Source: CAD feature listing. Evaluate the final solid. Frame: model axes, mm. A direction names the side the tool comes from. Give positions to 0.01 mm unless a question says otherwise; leave off trailing zeros. Write each loop counter-clockwise with the first axis right and the second up, starting at its lowest first coordinate (ties: lowest second). Pieces come first, ordered by that corner, then holes. Notation, with made-up numbers: (86.5, -35.75) -> (122.5, -35.75) arc R11 ccw to (122.5, -25.75) -> close; hole circle Ø3 at (35.5, -16). An arc over 180 degrees is marked (long way). Use a Markdown table: item, result. Add a question column.
```python
from build123d import *

# Parameters (mm, degrees)
EXTRUDE_1_DEPTH           = 25
SKETCH_4_R                = 2.5
EXTRUDE_2_DEPTH           = 7
M5X0_8_TAPPED_HOLE1_D     = 4.2
M5X0_8_TAPPED_HOLE1_DEPTH = 14
M5X0_8_TAPPED_HOLE1_TIP   = 1.2618073


with BuildPart() as part:
    # 草圖1 → 填料-伸長1 (new body)
    with BuildSketch(Plane.XY):
        Polygon((-2.020725942, 3.5), (-4.041451884, 0), (-2.020725942, -3.5), (2.020725942, -3.5), (4.041451884, 0), (2.020725942, 3.5), align=None)
    extrude(amount=EXTRUDE_1_DEPTH)

    # 草圖4 → 填料-伸長2 (add)
    with BuildSketch(Plane(origin=(0, 0, 0), x_dir=(-1, 0, 0), z_dir=(0, 0, -1))):
        Circle(SKETCH_4_R)
    extrude(amount=EXTRUDE_2_DEPTH)

    # M5x0.8 Tapped Hole1
    with Locations(Plane.XY.offset(25)):
        with Locations((0, 0)):
            Hole(M5X0_8_TAPPED_HOLE1_D / 2, depth=M5X0_8_TAPPED_HOLE1_DEPTH)
            with Locations((0, 0, -(M5X0_8_TAPPED_HOLE1_DEPTH + M5X0_8_TAPPED_HOLE1_TIP / 2))):  # 118° drill point
                Cone(0, M5X0_8_TAPPED_HOLE1_D / 2, M5X0_8_TAPPED_HOLE1_TIP, mode=Mode.SUBTRACT)


solid = part.part
```
(1) Access query for faces 1 (the flat face through (0, -3.5, 12)), 2 (the cylindrical face through (0.54, -2.44, -3.45)), 3 (the cylindrical face through (-2.003, 0.631, 17.902)). Directions: +Z, -Z, +X, -X, +Y, -Y. A direction counts if a zero-diameter tool reaches every point of the face in a straight line with its end or side. Return the directions, or none.
(2) Material intervals for L1, parallel to Y at x = 0, z = 16.25; L2, parallel to Z at x = -3, y = -1.75; L3, parallel to X at y = 1.25, z = 18.5, sorted ascending.
(3) Cut plane A-A on z = 16. Return the cut outline in (x, y), then the cut area to 3 significant figures.
(4) Cut plane B-B on z = -3. Return the cut outline in (x, y).
(5) First-contact query: pin 1 Ø1.5 at (y, z) = (-2, 10) entering from -X; pin 2 Ø3.5 at (x, y) = (0, 0) entering from +Z. Flat tips, straight axial feed; report the tip coordinate or a pass-through.
(6) Mould query, pull axis Y, two halves, no side actions, for faces 4 (the flat face through (-3, 1.8, 12.3)), 5 (the conical face through (0.35, 0.11, 9.96)), 6 (the flat face through (3, -1.8, 12.3)). Classes: +Y half, -Y half, draft (parallel to the pull), parting line (faces both ways), or undercut.
Output:
| question | item | result |
|---|---|---|
| 1 | face 1 | +Z, -Z, +X, -X, -Y |
| 1 | face 2 | -Z |
| 1 | face 3 | +Z |
| 2 | L1 | -3.5 to -2.1, 2.1 to 3.5 |
| 2 | L2 | 0 to 25 |
| 2 | L3 | -3.32 to -1.69, 1.69 to 3.32 |
| 3 | outline | (-4.04, 0) -> (-2.02, -3.5) -> (2.02, -3.5) -> (4.04, 0) -> (2.02, 3.5) -> (-2.02, 3.5) -> close; hole circle Ø4.2 at (0, 0) |
| 3 | area | 28.6 mm^2 |
| 4 | outline | circle Ø5 at (0, 0) |
| 5 | pin 1 | x = -3.32 |
| 5 | pin 2 | z = 10.79 |
| 6 | face 4 | +Y half |
| 6 | face 5 | undercut |
| 6 | face 6 | -Y half |
